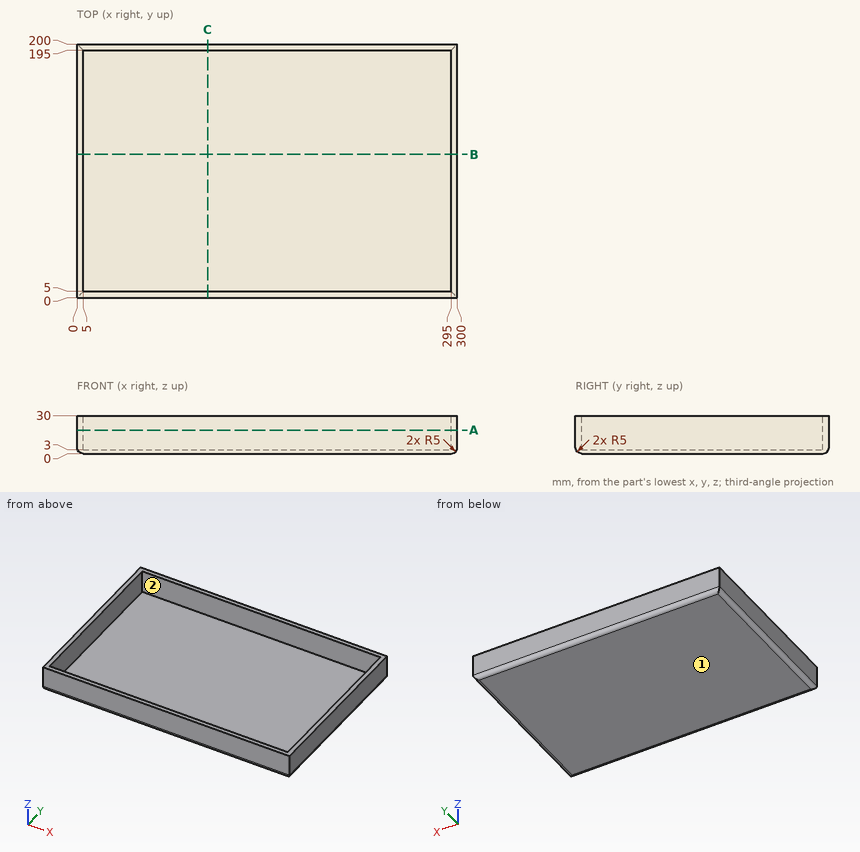
For this review, use the dimensioned drawing (mm, ordinates from the lowest corner) and the shaded views. A direction names the side the tool comes from. Give positions to 0.01 mm unless a question says otherwise; leave off trailing zeros. Order: outer loops, then holes, each group sorted by start corner. A loop starts at its lowest first (then second) coordinate and runs counter-clockwise, first axis right, second up. Notation, with made-up numbers: (-9.75, 57.5) -> (44.25, 57.5) arc R18 cw to (44.25, 71.5) -> close; hole circle Ø9 at (-14.75, 59.5). An arc over 180 degrees is marked (long way). Write item = value, one per line. Start each with the question number.
(1) Take a section at C-C (x = 103). Write out the cut boundary in (y, z), plus the area to 3 significant figures.
(2) For L1, parallel to Y at x = 17, z = 11; L2, parallel to X at y = 182, z = 12.25; L3, parallel to Z at x = 260.5, y = 119, list the stretches that pass through material, from the lowest coordinate up. Write a range as from..to.
(3) Take a section at A-A (z = 18.5). Write out the cut boundary in (x, y), plus the area to 3 significant figures.
(4) Tool access review of the marked faces 1 and 2: name each direction out of +Z, -Z, +X, -X, +Y, -Y from which nothing blocks a thin tool from reaching the whole face with its end or side.
(5) Take a section at B-B (y = 113). Write out the cut boundary in (x, z).
(6) For pin 1 Ø10 at (x, y) = (173, 161.5) entering from +Z, flat-tipped, find the tip position at first contact; note if it passes through.
Returned:
q1.outline = (0, 5) arc R5 ccw to (5, 0) -> (195, 0) arc R5 ccw to (200, 5) -> (200, 30) -> (195, 30) -> (195, 3) -> (5, 3) -> (5, 30) -> (0, 30) -> close
q1.area = 859 mm²
q2.L1 = 0..5, 195..200
q2.L2 = 0..5, 295..300
q2.L3 = 0..3
q3.outline = (0, 0) -> (300, 0) -> (300, 200) -> (0, 200) -> close; hole (5, 5) -> (295, 5) -> (295, 195) -> (5, 195) -> close
q3.area = 4,900 mm²
q4.face_1 = -Z, +X, -X, +Y, -Y
q4.face_2 = +Z
q5.outline = (0, 5) arc R5 ccw to (5, 0) -> (295, 0) arc R5 ccw to (300, 5) -> (300, 30) -> (295, 30) -> (295, 3) -> (5, 3) -> (5, 30) -> (0, 30) -> close
q6.pin_1 = 3
